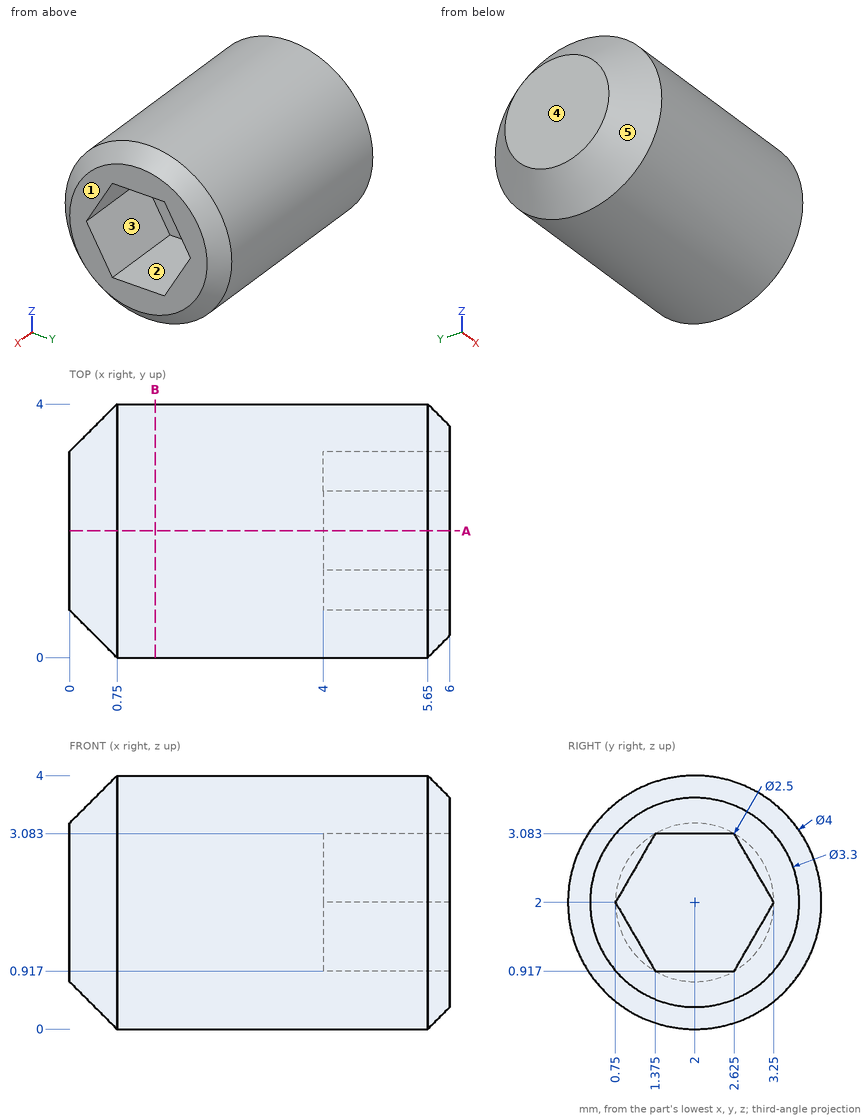
Answer from the drawing. Dimensions are ordinates in mm from the lowest x, y and z of the part. A direction names the side the tool comes from. Coordinates: 2 decimals unless noted, no trailing zeros. Write each loop counter-clockwise with the first axis right and the second up, starting at its lowest first coordinate (ties: lowest second). Pieces come first, ordered by that corner, then holes. Notation, with made-up numbers: M -24,-36.75 L 30,-36.75 A6 cw 30,-32.75 Z; hole C -4,-32.75 d6. An arc over 180 degrees is marked long. Write item = value, one per line.
1. Determine the mould class of the marked faces 3, 4 and 5 for opening direction Z: released by +Z, released by -Z, zero draft, split by the parting line, or undercut.
Solution:
face_3 = undercut
face_4 = zero draft
face_5 = split by the parting line
2. The part is cut by section A-A (y = 2). Determine the outline of the cut face in (x, z), then the cut area to 3 significant figures.
Solution:
outline = M 0,0.75 L 0.75,0 L 5.65,0 L 6,0.35 L 6,0.92 L 4,0.92 L 4,3.08 L 6,3.08 L 6,3.65 L 5.65,4 L 0.75,4 L 0,3.25 Z
area = 19.0 mm2
3. For the marked faces 1 and 2, determine the directions among +Z, -Z, +X, -X, +Y, -Y from which every point of the face is accessible in a straight line to the end or side of a thin tool.
Solution:
face_1 = +Z, -Z, +X, +Y, -Y
face_2 = +X
4. Straight lines are drawn through the part: line 1 (Y direction, x = 5.3, z = 3.05) (1 decimal); line 2 (Z direction, x = 1.25, y = 1.9); line 3 (Y direction, x = 2.8, z = 2.8). For each, find the intervals that lie inside material, in ascending order. Write a range as from..to.
Solution:
line_1 = 0.3..1.4, 2.6..3.7
line_2 = 0..4
line_3 = 0.17..3.83
5. The part is cut by section B-B (x = 1.35). Determine the outline of the cut face in (y, z), then the cut area to 3 significant figures.
Solution:
outline = C 2,2 d4
area = 12.6 mm2
